```python
from build123d import *

# Parameters (mm, degrees)
CUT_EXTRUDE1_DEPTH = 35


with BuildPart() as part:
    # Sketch1 → Revolve1 (revolve)
    with BuildSketch(Plane(origin=(0, 0, 0), x_dir=(0, 0, -1), z_dir=(1, 0, 0)), mode=Mode.PRIVATE) as revolve1_sk:
        Polygon((8, 0), (8, 6), (0, 6), (0, 32), (-30, 32), (-30, 0), align=None)
    revolve(revolve1_sk.sketch.rotate(Axis((0, 0, -8), (0, 0, -1)), 90), axis=Axis((0, 0, -8), (0, 0, -1)))

    # Sketch2 → Cut-Extrude1 (cut, symmetric)
    with BuildSketch(Plane(origin=(0, 0, 0), x_dir=(1, 0, 0), z_dir=(0, 1, 0))):
        with BuildLine():
            Line((-28.5, -30), (-2.5, -14.988893001))
            ThreePointArc((-2.5, -14.988893001), (0, -14.31902002), (2.5, -14.988893001))
            Line((2.5, -14.988893001), (28.5, -30))
            Line((28.5, -30), (-28.5, -30))
        make_face()
    extrude(amount=CUT_EXTRUDE1_DEPTH, both=True, mode=Mode.SUBTRACT)


solid = part.part
```
For this review, take the finished solid that the model builds, in its own axes (mm). A direction names the side the tool comes from. Round coordinates to 2 decimals unless told otherwise and drop trailing zeros. Write each loop counter-clockwise with the first axis right and the second up, starting at its lowest first coordinate (ties: lowest second). Pieces come first, ordered by that corner, then holes. Notation, with made-up numbers: (-9.75, 14.5) -> (21.25, 14.5) arc R10 cw to (21.25, 32.5) -> close; hole circle Ø1 at (38, -33). An arc over 180 degrees is marked (long way). One line per question, with ' | ' between items. Start each with the question number.
(1) For line 1 along X through (y, z) = (19, 21.5); line 2 along Y through (x, z) = (-28.5, 0.5); line 3 along Z through (x, y) = (1.5, 20.5), list the stretches that pass through material, from the lowest coordinate up. Write a range as from..to.
(2) Add section D-D, the plane z = 6.5. Write out the cut boundary in (x, y), plus the area to 3 significant figures.
(3) Add section C-C, the plane z = 22. Write out the cut boundary in (x, y), plus the area to 3 significant figures.
(4) Mouldability with a two-part tool opening along X and no side actions: class faces 1 (the face through (29.56, 12.26, 11.88)), 2 (the face through (-7, 0, 0)), 3 (the face through (-0.04, 0.45, 14.32)) as released by +X, released by -X, zero draft, split by the parting line, or undercut.
(5) Tool access review of faces 4 (the face through (5.723, -1.802, -3.944)), 5 (the face through (-12.79, 0.45, 20.93)), 6 (the face through (0, 0, -8)): name each direction out of +Z, -Z, +X, -X, +Y, -Y from which nothing blocks a thin tool from reaching the whole face with its end or side.
(6) Add section B-B, the plane x = 0. Write out the cut boundary in (y, z), plus the area to 3 significant figures.
(7) Insertion check: P1, Ø2, axis at x = 14, y = 1.5, coming from the -Z side; P2, Ø2, axis at y = -0.5, z = 6.5, coming from the +X side; P3, Ø6, axis at y = 25, z = 13.5, coming from the +X side; P4, Ø2, axis at y = 11.5, z = 23, coming from the -X side. Each pin has a flat end and moves straight along its axis. Give the tip position at first contact, or say it passes through.
(8) Add section A-A, the plane y = 0. Write out the cut boundary in (x, z).
Answer list:
1) line 1: -25.75..-13.78, 13.78..25.75 | line 2: -14.55..14.55 | line 3: 0..14.55
2) outline: circle Ø64 at (0, 0) | area: 3,220 mm²
3) outline: (-14.64, -28.45) -> (-14.64, 28.45) arc R32 ccw to start; (14.64, -28.45) arc R32 ccw to (14.64, 28.45) -> close | area: 1,410 mm²
4) face 1: split by the parting line | face 2: zero draft | face 3: undercut
5) face 4: -Z | face 5: +Z, +Y, -Y | face 6: -Z, +X, -X, +Y, -Y
6) outline: (-32, 0) -> (-6, 0) -> (-6, -8) -> (6, -8) -> (6, 0) -> (32, 0) -> (32, 14.32) -> (-32, 14.32) -> close | area: 1,010 mm²
7) P1: z = 0 | P2: x = 32 | P3: x = 23.24 | P4: x = -30.23
8) outline: (-32, 0) -> (-6, 0) -> (-6, -8) -> (6, -8) -> (6, 0) -> (32, 0) -> (32, 30) -> (28.5, 30) -> (2.5, 14.99) arc R5 cw to (-2.5, 14.99) -> (-28.5, 30) -> (-32, 30) -> close
